```python
from build123d import *

# Parameters (mm, degrees)
SKETCH1_W           = 63.627
SKETCH1_H           = 63.627
BOSS_EXTRUDE1_DEPTH = 2.7178
CUT_EXTRUDE1_DEPTH  = 0.762
SKETCH3_W           = 58.293
SKETCH3_H           = 58.293
BOSS_EXTRUDE2_DEPTH = 1.6002
SKETCH4_W           = 55.0926
SKETCH4_H           = 55.0926
CUT_EXTRUDE2_DEPTH  = 1.6002
SKETCH5_W           = 3.175
SKETCH5_H           = 1.6002
SKETCH6_W           = 3.175
SKETCH6_H           = 1.6002
SKETCH7_W           = 3.175
SKETCH7_H           = 1.6002
SKETCH8_W           = 3.175
SKETCH8_H           = 1.6002
FILLET1_R           = 7.9502
FILLET2_R           = 2.3876
FILLET3_R           = 3.683
FILLET4_R           = 5.2832


with BuildPart() as part:
    # Sketch1 → Boss-Extrude1 (new body)
    with BuildSketch(Plane(origin=(0, 0, 0), x_dir=(1, 0, 0), z_dir=(0, 1, 0))):
        Rectangle(SKETCH1_W, SKETCH1_H)
    extrude(amount=-BOSS_EXTRUDE1_DEPTH)

    # Sketch2 → Cut-Extrude1 (cut)
    with BuildSketch(Plane(origin=(0, 0, 0), x_dir=(-1, 0, 0), z_dir=(0, 1, 0))):
        Polygon((12.685676302, -28.8925), (28.8925, -12.685676302), (28.8925, 12.685676302), (12.685676302, 28.8925), (-12.685676302, 28.8925), (-28.8925, 12.685676302), (-28.8925, -12.685676302), (-12.685676302, -28.8925), align=None)
    extrude(amount=-CUT_EXTRUDE1_DEPTH, mode=Mode.SUBTRACT)

    # Sketch3 → Boss-Extrude2 (add)
    with BuildSketch(Plane.XZ.offset(2.7178)):
        Rectangle(SKETCH3_W, SKETCH3_H)
    extrude(amount=BOSS_EXTRUDE2_DEPTH)

    # Sketch4 → Cut-Extrude2 (cut)
    with BuildSketch(Plane.XZ.offset(4.318)):
        Rectangle(SKETCH4_W, SKETCH4_H)
    extrude(amount=-CUT_EXTRUDE2_DEPTH, mode=Mode.SUBTRACT)

    # Sketch5 → Revolve1 (revolve)
    with BuildSketch(Plane(origin=(0, 0, -23.6855), x_dir=(-1, 0, 0), z_dir=(0, 0, -1)), mode=Mode.PRIVATE) as revolve1_sk:
        with Locations((22.098, -3.5179)):
            Rectangle(SKETCH5_W, SKETCH5_H)
    revolve(revolve1_sk.sketch.rotate(Axis((-23.6855, -4.318, -23.6855), (0, 1, 0)), 270), axis=Axis((-23.6855, -4.318, -23.6855), (0, 1, 0)))

    # Sketch6 → Revolve2 (revolve)
    with BuildSketch(Plane(origin=(0, 0, 23.6855), x_dir=(-1, 0, 0), z_dir=(0, 0, -1)), mode=Mode.PRIVATE) as revolve2_sk:
        with Locations((-25.273, -3.5179)):
            Rectangle(SKETCH6_W, SKETCH6_H)
    revolve(revolve2_sk.sketch.rotate(Axis((23.6855, -4.318, 23.6855), (0, 1, 0)), 270), axis=Axis((23.6855, -4.318, 23.6855), (0, 1, 0)))

    # Sketch7 → Revolve3 (revolve)
    with BuildSketch(Plane(origin=(0, 0, 23.6855), x_dir=(-1, 0, 0), z_dir=(0, 0, -1)), mode=Mode.PRIVATE) as revolve3_sk:
        with Locations((22.098, -3.5179)):
            Rectangle(SKETCH7_W, SKETCH7_H)
    revolve(revolve3_sk.sketch.rotate(Axis((-23.6855, -4.318, 23.6855), (0, 1, 0)), 270), axis=Axis((-23.6855, -4.318, 23.6855), (0, 1, 0)))

    # Sketch8 → Revolve4 (revolve)
    with BuildSketch(Plane(origin=(0, 0, -23.6855), x_dir=(-1, 0, 0), z_dir=(0, 0, -1)), mode=Mode.PRIVATE) as revolve4_sk:
        with Locations((-25.273, -3.5179)):
            Rectangle(SKETCH8_W, SKETCH8_H)
    revolve(revolve4_sk.sketch.rotate(Axis((23.6855, -4.318, -23.6855), (0, 1, 0)), 270), axis=Axis((23.6855, -4.318, -23.6855), (0, 1, 0)))

    # Sketch9 → Cut-Revolve1 (revolve, cut)
    with BuildSketch(Plane.XY.offset(-23.6855), mode=Mode.PRIVATE) as cut_revolve1_sk:
        Polygon((-20.5994, 0), (-23.6855, 0), (-23.6855, -4.318), (-22.2123, -4.318), (-22.045796889, -2.414860733), (-20.672453944, -0.835010396), align=None)
    revolve(cut_revolve1_sk.sketch.rotate(Axis((-23.6855, 0, -23.6855), (0, -1, 0)), 270), axis=Axis((-23.6855, 0, -23.6855), (0, -1, 0)), mode=Mode.SUBTRACT)

    # Sketch10 → Cut-Revolve2 (revolve, cut)
    with BuildSketch(Plane.XY.offset(23.6855), mode=Mode.PRIVATE) as cut_revolve2_sk:
        Polygon((26.7716, 0), (23.6855, 0), (23.6855, -4.318), (25.1587, -4.318), (25.325203111, -2.414860733), (26.698546056, -0.835010396), align=None)
    revolve(cut_revolve2_sk.sketch.rotate(Axis((23.6855, 0, 23.6855), (0, -1, 0)), 270), axis=Axis((23.6855, 0, 23.6855), (0, -1, 0)), mode=Mode.SUBTRACT)

    # Sketch11 → Cut-Revolve3 (revolve, cut)
    with BuildSketch(Plane.XY.offset(23.6855), mode=Mode.PRIVATE) as cut_revolve3_sk:
        Polygon((-20.5994, 0), (-23.6855, 0), (-23.6855, -4.318), (-22.2123, -4.318), (-22.045796889, -2.414860733), (-20.672453944, -0.835010396), align=None)
    revolve(cut_revolve3_sk.sketch.rotate(Axis((-23.6855, 0, 23.6855), (0, -1, 0)), 270), axis=Axis((-23.6855, 0, 23.6855), (0, -1, 0)), mode=Mode.SUBTRACT)

    # Sketch12 → Cut-Revolve4 (revolve, cut)
    with BuildSketch(Plane.XY.offset(-23.6855), mode=Mode.PRIVATE) as cut_revolve4_sk:
        Polygon((26.7716, 0), (23.6855, 0), (23.6855, -4.318), (25.1587, -4.318), (25.325203111, -2.414860733), (26.698546056, -0.835010396), align=None)
    revolve(cut_revolve4_sk.sketch.rotate(Axis((23.6855, 0, -23.6855), (0, -1, 0)), 270), axis=Axis((23.6855, 0, -23.6855), (0, -1, 0)), mode=Mode.SUBTRACT)

    # Fillet1
    fillet1_edges = [part.edges().sort_by_distance(p)[0] for p in [
        (31.8135, -1.3589, 31.8135),
        (-31.8135, -1.3589, 31.8135),
        (-31.8135, -1.3589, -31.8135),
        (31.8135, -1.3589, -31.8135),
    ]]
    fillet(fillet1_edges, radius=FILLET1_R)

    # Fillet2
    fillet2_edges = [part.edges().sort_by_distance(p)[0] for p in [
        (0, 0, 31.8135),
        (31.8135, 0, 0),
        (0, 0, -31.8135),
        (-31.8135, 0, 0),
        (29.484940332, 0, -29.484940332),
        (-29.484940332, 0, 29.484940332),
        (-29.484940332, 0, -29.484940332),
        (29.484940332, 0, 29.484940332),
        (-12.685676302, -0.381, -28.8925),
        (12.685676302, -0.381, -28.8925),
        (28.8925, -0.381, -12.685676302),
        (28.8925, -0.381, 12.685676302),
        (12.685676302, -0.381, 28.8925),
        (-12.685676302, -0.381, 28.8925),
        (-28.8925, -0.381, 12.685676302),
        (-28.8925, -0.381, -12.685676302),
    ]]
    fillet(fillet2_edges, radius=FILLET2_R)

    # Fillet3
    fillet3_edges = [part.edges().sort_by_distance(p)[0] for p in [
        (-27.5463, -3.5179, -27.5463),
        (-27.5463, -3.5179, 27.5463),
        (27.5463, -3.5179, 27.5463),
        (27.5463, -3.5179, -27.5463),
    ]]
    fillet(fillet3_edges, radius=FILLET3_R)

    # Fillet4
    fillet4_edges = [part.edges().sort_by_distance(p)[0] for p in [
        (29.1465, -3.5179, -29.1465),
        (29.1465, -3.5179, 29.1465),
        (-29.1465, -3.5179, 29.1465),
        (-29.1465, -3.5179, -29.1465),
    ]]
    fillet(fillet4_edges, radius=FILLET4_R)


solid = part.part
```
Source: CAD feature listing. Evaluate the final solid. Frame: model axes, mm. A direction names the side the tool comes from. Give positions to 0.01 mm unless a question says otherwise; leave off trailing zeros. Write each loop counter-clockwise with the first axis right and the second up, starting at its lowest first coordinate (ties: lowest second). Pieces come first, ordered by that corner, then holes.
1. Section query B-B (x = 5). Return the cut outline in (y, z).
2. Access query for faces 1 (the face through (23.825, -3.507, -26.857)), 2 (the face through (29.146, -4, 0)), 3 (the face through (-27.6, -3.5, 27.6)). Directions: +Z, -Z, +X, -X, +Y, -Y. A direction counts if a zero-diameter tool reaches every point of the face in a straight line with its end or side. Return the directions, or none.
3. Section query A-A (z = -0.5). Return the cut outline in (x, y), then the cut area to 3 significant figures.
4. Material intervals for line 1 along X through (y, z) = (-0.6, 23); line 2 along X through (y, z) = (-2.9, 0.5); line 3 along X through (y, z) = (-3.9, -25.5), sorted ascending.
5. Pull-direction query (X, two-part tool) for faces 4 (the face through (0, -4, -27.546)), 5 (the face through (20.69, -0.38, 20.89)), 6 (the face through (31.096, -0.681, -0.334)), 7 (the face through (-29.55, -2.56, -29.42)); classes: +X half, -X half, draft (parallel to the pull), parting line (faces both ways), or undercut.
6. First-contact query: pin 1 (2 mm diameter, centred on x = -19, z = 18.5, fed in from +Y); pin 2 (0.5 mm diameter, centred on y = -3.5, z = 4.5, fed in from +X); pin 3 (0.8 mm diameter, centred on x = -7.5, y = -3.5, fed in from -Z). Flat tips, straight axial feed; report the tip coordinate or a pass-through.
Output values:
1. outline: (-4.32, -29.15) - (-2.72, -29.15) - (-2.72, -31.81) - (-2.39, -31.81) arc R2.39 ccw to (0, -29.43) - (0, -28.89) - (-0.76, -28.89) - (-0.76, 28.89) - (0, 28.89) - (0, 29.43) arc R2.39 ccw to (-2.39, 31.81) - (-2.72, 31.81) - (-2.72, 29.15) - (-4.32, 29.15) - (-4.32, 27.55) - (-2.72, 27.55) - (-2.72, -27.55) - (-4.32, -27.55) - close
2. face 1: -Y
2. face 2: +Z, -Z, +X, -Y
2. face 3: +Z, -X, -Y
3. outline: (-31.81, -2.72) - (-29.15, -2.72) - (-29.15, -4.32) - (-27.55, -4.32) - (-27.55, -2.72) - (27.55, -2.72) - (27.55, -4.32) - (29.15, -4.32) - (29.15, -2.72) - (31.81, -2.72) - (31.81, -2.39) arc R2.39 ccw to (29.43, 0) - (28.89, 0) - (28.89, -0.76) - (-28.89, -0.76) - (-28.89, 0) - (-29.43, 0) arc R2.39 ccw to (-31.81, -2.39) - close
3. area: 132 mm2
4. line 1: x = -31.01 to -26.64, -20.73 to -18.58, 18.58 to 20.73, 26.64 to 31.01
4. line 2: x = -29.15 to -27.55, 27.55 to 29.15
4. line 3: x = -28.89 to -27.16, -26.29 to -21.08, 21.08 to 26.29, 27.16 to 28.89
5. face 4: undercut
5. face 5: undercut
5. face 6: +X half
5. face 7: -X half
6. pin 1: stops at y = -0.76
6. pin 2: stops at x = 29.15
6. pin 3: stops at z = -29.15
